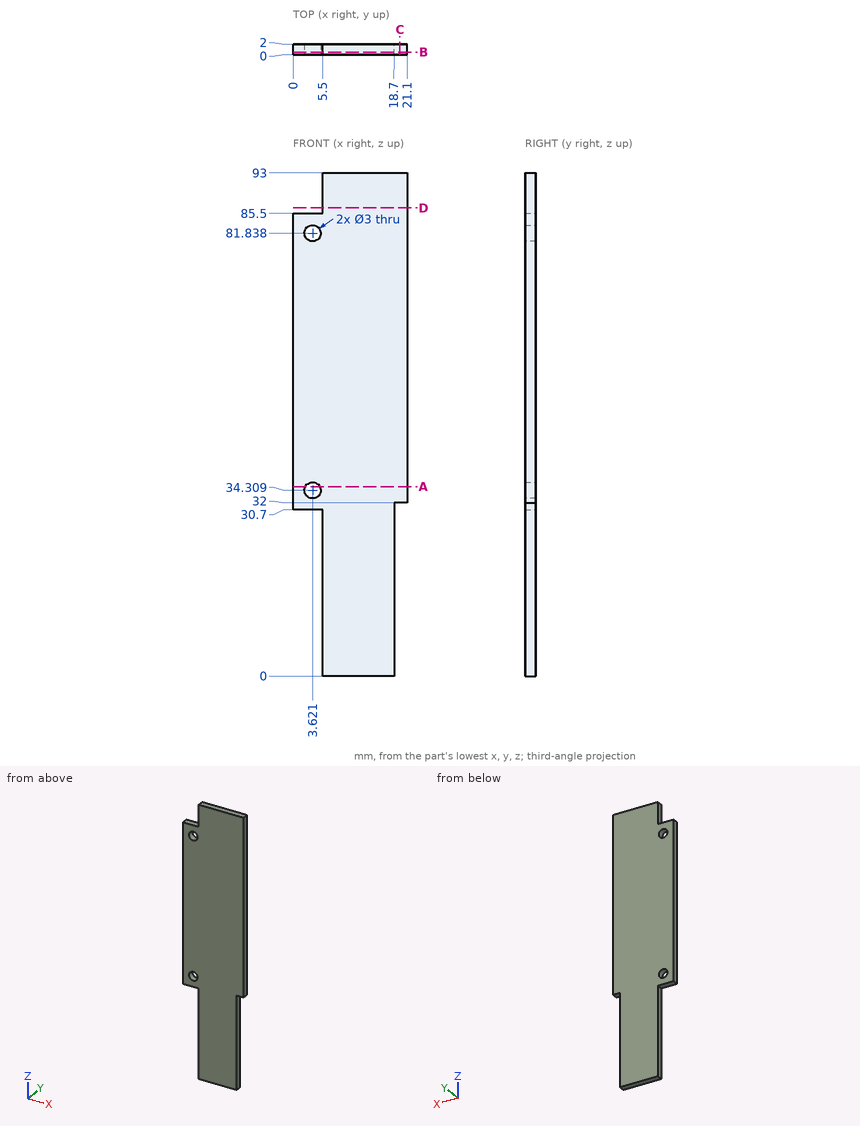
Part print with two shaded views. Sizes in mm from the minimum x, y, z corner. Coordinates: 2 decimals unless noted, no trailing zeros. Order: outer loops, then holes, each group sorted by start corner. A loop starts at its lowest first (then second) coordinate and runs counter-clockwise, first axis right, second up. Notation, with made-up numbers: (-38, -7.75) - (7, -7.75) arc R20 ccw to (7, 1.25) - close; hole circle Ø1 at (-9, -22.5). An arc over 180 degrees is marked (long way). Write item = value, one per line. Start each with the question number.
1) Saw through at B-B on y = 0.5. Write the cut outline in (x, z).
2) Flat gauge pins, fed straight in: pin 1 Ø1 at (y, z) = (1, 18) entering from -X; pin 2 Ø0.6 at (x, y) = (3.5, 1) entering from -Z; pin 3 Ø0.6 at (x, y) = (20, 1.5) entering from -Z. Where does each tip first touch, or does it go through?
3) Saw through at C-C on x = 19.75. Write the cut outline in (y, z).
4) Saw through at A-A on z = 35. Write the cut outline in (x, y).
5) Wall check: line 1 along Z through (x, y) = (3.5, 1); line 2 along Z through (x, y) = (2.75, 1.25) (1 decimal); line 3 along X through (y, z) = (0.85, 6.5). Give the ranges that are in metal, low to high. Write a range as from..to.
6) Saw through at D-D on z = 86.5. Write the cut outline in (x, y), then the cut area to 3 significant figures.
From the geometry:
q1.outline = (0, 30.7) - (5.5, 30.7) - (5.5, 0) - (18.7, 0) - (18.7, 32) - (21.1, 32) - (21.1, 93) - (5.5, 93) - (5.5, 85.5) - (0, 85.5) - close; hole circle Ø3 at (3.62, 34.31); hole circle Ø3 at (3.62, 81.84)
q2.pin_1 = 5.5
q2.pin_2 = 30.7
q2.pin_3 = 32
q3.outline = (0, 32) - (2, 32) - (2, 93) - (0, 93) - close
q4.outline = (0, 0) - (2.29, 0) - (2.29, 2) - (0, 2) - close; (4.95, 0) - (21.1, 0) - (21.1, 2) - (4.95, 2) - close
q5.line_1 = 30.7..32.81, 35.8..80.34, 83.33..85.5
q5.line_2 = 30.7..33.1, 35.5..80.6, 83.1..85.5
q5.line_3 = 5.5..18.7
q6.outline = (5.5, 0) - (21.1, 0) - (21.1, 2) - (5.5, 2) - close
q6.area = 31.2 mm^2
